Input: part model. Units: mm. Frame: model coordinates. Round coordinates to 2 decimals unless told otherwise and drop trailing zeros. Loops run counter-clockwise (first coordinate to the right, second up) from the corner with the lowest first, then second, coordinate; pieces in that order, holes last. Notation, with made-up numbers: M 55.25,0 L 95.25,0 A26 cw 95.25,39 Z; hole C -22,-23.5 d4. An arc over 180 degrees is marked long. Put each result on its own line as item: value. Start each with the question number.
1) Section B-B on x = 13. Output: boundary loops of the cut face in (y, z), plus the area to 3 significant figures.
2) Section C-C on y = -27.94. Output: boundary loops of the cut face in (x, z) (3 decimals).
3) Section A-A on y = -9. Output: boundary loops of the cut face in (x, z).
4) Line query: probe 1 along Y at (x, z) = (34.29, 0.75) (3 decimals); probe 2 along Y at (x, z) = (39.37, 0.7) (3 decimals); probe 3 along Y at (x, z) = (42, 2.35). Output: solid intervals per line, ascending.
5) Section D-D on z = 1.95. State how many separate pieces and enclosed holes the cut face has, plus the area to 3 significant figures.
6) Pin query (flat end, axial travel): pin 1 (6 mm diameter, centred on x = 33.5, y = -18.5, fed in from -Z); pin 2 (1.3 mm diameter, centred on y = -82.5, z = 1.5, fed in from -X). Return the tip coordinate at first contact, or that it passes through.
from build123d import *

# Parameters (mm, degrees)
BOSS_EXTRUDE1_DEPTH = 2.54
SKETCH4_R           = 1.905
SKETCH4_W           = 20.32
SKETCH4_H           = 50.8
CUT_EXTRUDE2_DEPTH  = 25.4
SKETCH5_W           = 20.32
SKETCH5_H           = 7.493
CUT_EXTRUDE3_DEPTH  = 5.08
SKETCH6_R           = 1.27
CUT_EXTRUDE4_DEPTH  = 5.08
SKETCH8_W           = 12.7
SKETCH8_H           = 2.54
SKETCH8_W_2         = 2.54
SKETCH8_H_2         = 12.7
CUT_EXTRUDE5_DEPTH  = 5.08


with BuildPart() as part:
    # Sketch1 → Boss-Extrude1 (new body)
    with BuildSketch(Plane.XY):
        Polygon((-4.120444444, 6.35), (53.34, 6.35), (53.34, -95.25), (16.22499019, -95.25), (-16.356614113, -78.274710363), (-26.416, -57.15), align=None)
    extrude(amount=BOSS_EXTRUDE1_DEPTH)

    # Sketch4 → Cut-Extrude2 (cut)
    with BuildSketch(Plane(origin=(0, 0, 0), x_dir=(-1, 0, 0), z_dir=(0, 0, -1))):
        with Locations((-39.37, -17.78)):
            Circle(SKETCH4_R)
        with Locations((-34.29, -17.78)):
            Circle(SKETCH4_R)
        with Locations((-39.37, -27.94)):
            Circle(SKETCH4_R)
        with Locations((-34.29, -27.94)):
            Circle(SKETCH4_R)
        with Locations((-41.91, -45.72)):
            Circle(SKETCH4_R)
        with Locations((-36.83, -45.72)):
            Circle(SKETCH4_R)
        with Locations((-44.45, -64.77)):
            Circle(SKETCH4_R)
        with Locations((-39.37, -64.77)):
            Circle(SKETCH4_R)
        with Locations((-44.45, -83.82)):
            Circle(SKETCH4_R)
        with Locations((-39.37, -83.82)):
            Circle(SKETCH4_R)
        with Locations((-24.257, -17.78)):
            Circle(SKETCH4_R)
        with Locations((-19.939, -17.78)):
            Circle(SKETCH4_R)
        with Locations((-24.257, -27.94)):
            Circle(SKETCH4_R)
        with Locations((-19.939, -27.94)):
            Circle(SKETCH4_R)
        with Locations((-26.162, -45.72)):
            Circle(SKETCH4_R)
        with Locations((-21.082, -45.72)):
            Circle(SKETCH4_R)
        with Locations((-27.686, -64.77)):
            Circle(SKETCH4_R)
        with Locations((-22.606, -64.77)):
            Circle(SKETCH4_R)
        with Locations((-7.62, -26.543)):
            Rectangle(SKETCH4_W, SKETCH4_H)
    extrude(amount=-CUT_EXTRUDE2_DEPTH, mode=Mode.SUBTRACT)

    # Sketch5 → Cut-Extrude3 (cut)
    with BuildSketch(Plane.XY.offset(2.54)):
        with Locations((7.62, 2.6035)):
            Rectangle(SKETCH5_W, SKETCH5_H)
    extrude(amount=-CUT_EXTRUDE3_DEPTH, mode=Mode.SUBTRACT)

    # Sketch6 → Cut-Extrude4 (cut)
    with BuildSketch(Plane.XY.offset(2.54)):
        with Locations((1.6002, -2.4384)):
            Circle(SKETCH6_R)
        with Locations((44.2976, -2.4384)):
            Circle(SKETCH6_R)
        with Locations((-17.4498, -57.15)):
            Circle(SKETCH6_R)
        with Locations((-10.5918, -71.3486)):
            Circle(SKETCH6_R)
        with Locations((18.796, -86.5378)):
            Circle(SKETCH6_R)
    extrude(amount=-CUT_EXTRUDE4_DEPTH, mode=Mode.SUBTRACT)

    # Sketch8 → Cut-Extrude5 (cut)
    with BuildSketch(Plane.XY.offset(2.54)):
        with Locations((29.972, -84.5566)):
            Rectangle(SKETCH8_W, SKETCH8_H)
        with Locations((20.066, -78.359)):
            Rectangle(SKETCH8_W_2, SKETCH8_H_2)
        with Locations((13.208, -81.026)):
            Rectangle(SKETCH8_W_2, SKETCH8_H_2)
        with Locations((5.588, -78.486)):
            Rectangle(SKETCH8_W_2, SKETCH8_H_2)
    extrude(amount=-CUT_EXTRUDE5_DEPTH, mode=Mode.SUBTRACT)


solid = part.part
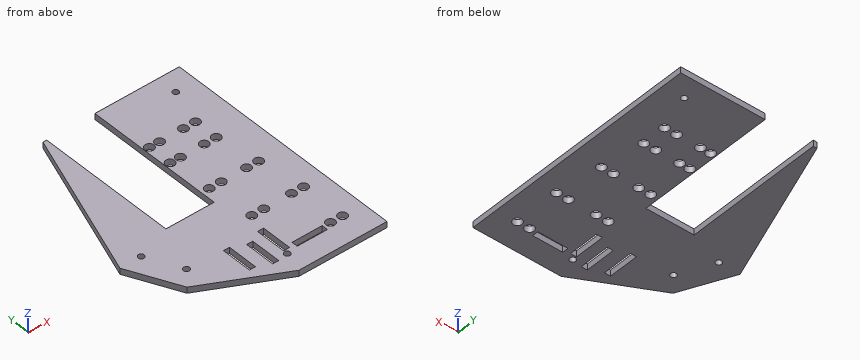
Geometry results:
1. outline: M -93.57,0 L -87.38,0 L -87.38,2.54 L -93.57,2.54 Z; M -74.68,0 L -51.94,0 L -51.94,2.54 L -74.68,2.54 Z
1. area: 73.5 mm²
2. outline: M -16.16,0 L -2.54,0 L -2.54,2.54 L -16.16,2.54 Z; M 17.78,0 L 18.034,0 L 18.034,2.54 L 17.78,2.54 Z; M 21.844,0 L 22.352,0 L 22.352,2.54 L 21.844,2.54 Z; M 26.162,0 L 32.385,0 L 32.385,2.54 L 26.162,2.54 Z; M 36.195,0 L 37.465,0 L 37.465,2.54 L 36.195,2.54 Z; M 41.275,0 L 53.34,0 L 53.34,2.54 L 41.275,2.54 Z
3. outline: M -9.51,0 L -2.54,0 L -2.54,2.54 L -9.51,2.54 Z; M 17.78,0 L 53.34,0 L 53.34,2.54 L 17.78,2.54 Z
4. probe 1: y = -95.25 to -85.827, -83.287 to -29.845, -26.035 to -19.685, -15.875 to 6.35
4. probe 2: y = -95.25 to -85.725, -81.915 to -66.675, -62.865 to -29.845, -26.035 to -19.685, -15.875 to 6.35
4. probe 3: y = -95.25 to -47.62, -43.82 to 6.35
5. separate pieces: 1
5. enclosed holes: 26
5. area: 5,300 mm²
6. pin 1: stops at z = 0
6. pin 2: stops at x = -9.49
